Model file for the job. Use its own axes, mm. Face numbers are marked on the shaded views. Round coordinates to 2 decimals unless told otherwise and drop trailing zeros. Order: outer loops, then holes, each group sorted by start corner. A loop starts at its lowest first (then second) coordinate and runs counter-clockwise, first axis right, second up. Notation, with made-up numbers: (-13, 50.25) - (41, 50.25) arc R19 ccw to (41, 75.25) - close; hole circle Ø1 at (49.25, 45). An arc over 180 degrees is marked (long way). Answer as CSV lines item,"result". Start each with the question number.
1. Wall check: line 1 along Z through (x, y) = (-7.5, -7); line 2 along X through (y, z) = (9, 26); line 3 along X through (y, z) = (18, 31.5). Give the ranges that are in metal, low to high. Write a range as [from, to].
2. Pin check, flat tips, straight feed: pin 1 Ø10 at (x, y) = (29.5, -23.5) entering from +Z; pin 2 Ø22.5 at (x, y) = (-11, 0.5) entering from +Z; pin 3 Ø6 at (x, z) = (-17, 21) entering from -Y. Stop position of each tip, or through.
3. Band-saw the part on C-C on z = 29. List the corners of the cut face in (x, y), then the cut area to 3 significant figures.
4. Band-saw the part on D-D on z = 5. List the corners of the cut face in (x, y).
5. Band-saw the part on A-A on y = 0. List the corners of the cut face in (x, z).
6. Pull direction Y, two halves, no side cores. Call the marked faces 1, 2, 3 and 4: released by +Y, released by -Y, zero draft, split by the parting line, or undercut.
```python
from build123d import *

# Parameters (mm, degrees)
F0_R     = 37.5
F1_DEPTH = 35
F3_R     = 22.5
F4_DEPTH = 10


# Not quite as in the source:
# - a fillet or chamfer that OpenCascade refuses, or shapes differently, is made with other operations: its cross-section is extruded or revolved along the edge and cut away or added


with BuildPart() as f1:
    # F0 (on Top) → F1 (new body)
    with BuildSketch(Plane.XY):
        Circle(F0_R)
    extrude(amount=F1_DEPTH)

    # F2: chamfer of 10 x 12 on 1 edges, made by hand

    # F2_s1 → F2_t2 (revolve, cut)
    with BuildSketch(Plane.XZ):
        Polygon((37.5, 23), (27.5, 35), (37.5, 35), align=None)
    revolve(axis=Axis((0, 0, 35), (0, 0, 1)), mode=Mode.SUBTRACT)

    # F3 (on face) → F4 (cut)
    with BuildSketch(Plane.XY.offset(35)):
        Circle(F3_R)
    extrude(amount=-F4_DEPTH, mode=Mode.SUBTRACT)

    # F5: chamfer of 10 on 2 edges, made by hand


with BuildPart() as f5_tool2:
    # F5_s3 → F5_t4 (revolve)
    with BuildSketch(Plane.XZ):
        Polygon((32.5, 35), (22.5, 25), (22.5, 35), align=None)
    revolve(axis=Axis((0, 0, 35), (0, 0, 1)))

    split(bisect_by=Plane.XY.offset(25), keep=Keep.TOP)


with BuildPart() as f1_1:
    add(f1.part)

    # F5_t1: cut F5_tool2
    add(f5_tool2.part, mode=Mode.SUBTRACT)

    # F5_s6 → F5_t7 (revolve, cut)
    with BuildSketch(Plane.XZ):
        Polygon((37.5, 10), (27.5, 0), (37.5, 0), align=None)
    revolve(axis=Axis((0, 0, 0), (0, 0, 1)), mode=Mode.SUBTRACT)


solid = f1_1.part
```
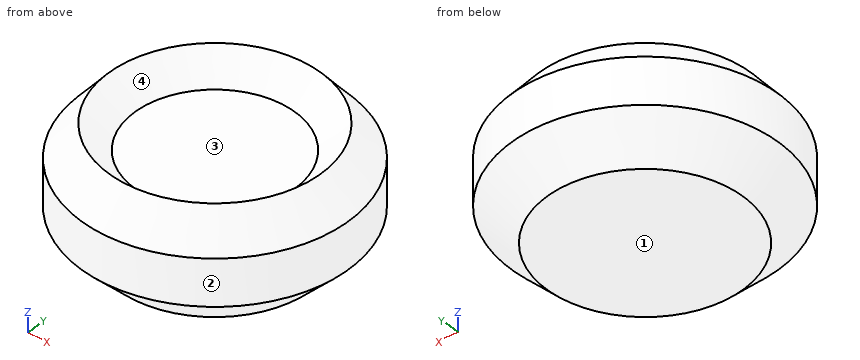
Reply:
1,line 1,"z = [0, 25]"
1,line 2,"x = [-33.82, -21.71], [21.71, 33.82]"
1,line 3,"x = [-24.52, -22.74], [22.74, 24.52]"
2,pin 1,"stops at z = 28.74"
2,pin 2,"stops at z = 25"
2,pin 3,"stops at y = -34.79"
3,outline,"circle Ø65 at (0, 0); hole circle Ø53 at (0, 0)"
3,area,"1,110 mm2"
4,outline,"circle Ø65 at (0, 0)"
5,outline,"(-37.5, 10) - (-27.5, 0) - (27.5, 0) - (37.5, 10) - (37.5, 23) - (29.77, 32.27) - (22.5, 25) - (-22.5, 25) - (-29.77, 32.27) - (-37.5, 23) - close"
6,face 1,"zero draft"
6,face 2,"split by the parting line"
6,face 3,"undercut"
6,face 4,"undercut"
